```python
from build123d import *

# Parameters (mm, degrees)
BOSS_EXTRUDE1_DEPTH = 1.6


with BuildPart() as part:
    # Sketch1 → Boss-Extrude1 (new body)
    with BuildSketch(Plane(origin=(0, -12.08184695, 0), x_dir=(1, 0, 0), z_dir=(0, 1, 0))):
        with BuildLine():
            Line((7.068263687, 41.600601737), (-7.059496612, 41.600601737))
            ThreePointArc((-7.059496612, 41.600601737), (-8.738121808, 40.953226214), (-9.547386312, 39.346375699))
            add(Edge.make_bspline(
                [(-9.547386312, 39.346375699), (-9.791801042, 36.872209768), (-10.174780597, 34.427308106), (-11.191257392, 29.590412993), (-11.825986881, 27.198679788), (-13.350641046, 22.469109457), (-14.231234092, 20.161687267), (-16.219413971, 15.670679569), (-17.327255507, 13.484910955), (-19.77160384, 9.233454443), (-21.107913128, 7.167662826), (-23.287017843, 4.160685833), (-24.044102201, 3.171933948), (-25.600832941, 1.24516113), (-26.401965146, 0.30483539), (-30.518180843, -4.284811803), (-34.16377144, -7.599360565), (-38.1299904, -10.589142877)],
                knots=[0, 0, 0, 0, 0.125, 0.125, 0.25, 0.25, 0.375, 0.375, 0.5, 0.5, 0.625, 0.625, 0.6875, 0.6875, 0.75, 0.75, 1, 1, 1, 1], degree=3))
            ThreePointArc((-38.1299904, -10.589142877), (-39.094420308, -12.194619809), (-38.673009405, -14.019474345))
            ThreePointArc((-38.673009405, -14.019474345), (-38.081769626, -16.566513233), (-39.42061036, -18.812503006))
            ThreePointArc((-39.42061036, -18.812503006), (-40.390492541, -20.517035077), (-39.831968266, -22.396969027))
            add(Edge.make_bspline(
                [(-39.831968266, -22.396969027), (-38.283172708, -24.266437753), (-36.643071519, -26.058655413), (-33.174318098, -29.455880725), (-31.352030623, -31.054807711), (-29.43071323, -32.539448808)],
                knots=[0, 0, 0, 0, 0.5, 0.5, 1, 1, 1, 1], degree=3))
            add(Edge.make_bspline(
                [(-29.43071323, -32.539448808), (-27.320643605, -34.16992841), (-25.110907511, -35.649716155), (-20.460386406, -38.259954595), (-18.045119378, -39.375356082), (-14.281591244, -40.731351728), (-13.014141837, -41.126537478), (-10.462616624, -41.801653768), (-9.177088412, -42.082104136), (-5.291542564, -42.754094477), (-2.662588178, -42.976416738), (0.004383999, -42.976416738)],
                knots=[0, 0, 0, 0, 0.25, 0.25, 0.5, 0.5, 0.625, 0.625, 0.75, 0.75, 1, 1, 1, 1], degree=3))
            add(Edge.make_bspline(
                [(0.004383999, -42.976416738), (2.671656674, -42.976416738), (5.319285582, -42.754113953), (9.259525556, -42.067540092), (10.556225677, -41.781619701), (13.107012662, -41.101381696), (14.362802441, -40.706759914), (16.836410325, -39.811946458), (18.054248498, -39.311810579), (20.452976989, -38.208815379), (21.635192506, -37.605209835), (25.119535884, -35.649249598), (27.327228533, -34.170936704), (29.435499854, -32.542167102)],
                knots=[0, 0, 0, 0, 0.25, 0.25, 0.375, 0.375, 0.5, 0.5, 0.625, 0.625, 0.75, 0.75, 1, 1, 1, 1], degree=3))
            add(Edge.make_bspline(
                [(29.435499854, -32.542167102), (31.356661411, -31.057999079), (33.183178175, -29.455634698), (36.651766782, -26.058931244), (38.289020033, -24.270113959), (39.837842074, -22.401078618)],
                knots=[0, 0, 0, 0, 0.5, 0.5, 1, 1, 1, 1], degree=3))
            ThreePointArc((39.837842074, -22.401078618), (40.396592097, -20.52122374), (39.426929699, -18.816579853))
            ThreePointArc((39.426929699, -18.816579853), (38.088433126, -16.570796705), (38.67950123, -14.024082445))
            ThreePointArc((38.67950123, -14.024082445), (39.100802356, -12.199274218), (38.136401576, -10.593861236))
            add(Edge.make_bspline(
                [(38.136401576, -10.593861236), (34.168623759, -7.602959081), (30.509352448, -4.27682522), (26.366767099, 0.349726066), (25.563654335, 1.294607123), (24.01416015, 3.216210378), (23.26679186, 4.194046735), (21.106661228, 7.178559095), (19.77567512, 9.236115194), (17.332454935, 13.487332018), (16.22037441, 15.681088283), (14.719864957, 19.076008242), (14.246709963, 20.227996379), (13.365900278, 22.544460809), (12.957352394, 23.710625613), (11.82518653, 27.232396594), (11.194571791, 29.611161178), (10.183276163, 34.430925487), (9.800625177, 36.871434644), (9.556155738, 39.346351897)],
                knots=[0, 0, 0, 0, 0.25, 0.25, 0.3125, 0.3125, 0.375, 0.375, 0.5, 0.5, 0.625, 0.625, 0.6875, 0.6875, 0.75, 0.75, 0.875, 0.875, 1, 1, 1, 1], degree=3))
            ThreePointArc((9.556155738, 39.346351897), (8.746897744, 40.953218184), (7.068263687, 41.600601737))
        make_face()
        with BuildLine():
            ThreePointArc((2.917114338, 9.477212595), (2.756374668, 5.872981189), (3.951101823, 2.468726748))
            add(Edge.make_bspline(
                [(18.704113686, -16.363172993), (17.992145269, -15.660180667), (17.284020826, -14.953500566), (15.898077439, -13.511066303), (15.216988025, -12.778449721), (13.209804316, -10.545981706), (11.922619235, -9.014699706), (8.217020706, -4.29052926), (5.969838206, -0.988031562), (3.951101823, 2.468726748)],
                knots=[0, 0, 0, 0, 0.125, 0.125, 0.25, 0.25, 0.5, 0.5, 1, 1, 1, 1], degree=3))
            ThreePointArc((18.704113686, -16.363172993), (19.293025471, -17.93950559), (18.470275007, -19.407403142))
            add(Edge.make_bspline(
                [(-18.494716896, -19.382200256), (-18.156747928, -19.627153591), (-17.818664146, -19.871886584), (-17.13548839, -20.34790294), (-16.790775019, -20.579912893), (-15.746956693, -21.257369006), (-15.038196301, -21.684285132), (-12.870713002, -22.885961299), (-11.370716058, -23.581511117), (-9.025130071, -24.441385157), (-8.223466165, -24.698129558), (-6.613792479, -25.137565491), (-5.80401834, -25.321234472), (-3.359849379, -25.763841436), (-1.710600897, -25.914327465), (0.793635304, -25.91836178), (1.634808791, -25.88219159), (3.293827112, -25.736118011), (4.115824788, -25.626398759), (6.559865603, -25.190037003), (8.159961985, -24.756217145), (10.518010173, -23.899908948), (11.293937095, -23.580881464), (12.808242427, -22.888006864), (13.549502528, -22.513052805), (15.00267183, -21.710479018), (15.714628815, -21.282945031), (16.762116652, -20.60495391), (17.107865076, -20.372830636), (17.792765058, -19.896747026), (18.131563633, -19.652153318), (18.470275007, -19.407403142)],
                knots=[0, 0, 0, 0, 0.03125, 0.03125, 0.0625, 0.0625, 0.125, 0.125, 0.25, 0.25, 0.3125, 0.3125, 0.375, 0.375, 0.5, 0.5, 0.5625, 0.5625, 0.625, 0.625, 0.75, 0.75, 0.8125, 0.8125, 0.875, 0.875, 0.9375, 0.9375, 0.96875, 0.96875, 1, 1, 1, 1], degree=3))
            ThreePointArc((-18.494716896, -19.382200256), (-19.313315476, -17.938131693), (-18.759498896, -16.373291495))
            add(Edge.make_bspline(
                [(-4.019478984, 2.418815751), (-6.073388857, -1.004555589), (-8.371219964, -4.274194721), (-12.087144101, -8.96897705), (-13.369226154, -10.496572825), (-15.349259798, -12.736872688), (-16.018851728, -13.47516887), (-17.376233604, -14.935672121), (-18.066404983, -15.655773734), (-18.759498896, -16.373291495)],
                knots=[0, 0, 0, 0, 0.5, 0.5, 0.75, 0.75, 0.875, 0.875, 1, 1, 1, 1], degree=3))
            ThreePointArc((-4.019478984, 2.418815751), (-2.778667962, 5.846147783), (-2.919787203, 9.488441319))
            ThreePointArc((-2.919787203, 9.488441319), (0.005771232, 13.17752407), (2.917114338, 9.477212595))
        make_face(mode=Mode.SUBTRACT)
    extrude(amount=BOSS_EXTRUDE1_DEPTH)


solid = part.part
```
CAD build for the part. Positions are in the model's coordinates, mm. Round coordinates to 2 decimals unless told otherwise and drop trailing zeros. One line per question, with ' | ' between items.
Q1. Drop a flat-ended pin along its axis: pin 1 (7 mm diameter, centred on x = 0, z = -10.18, fed in from +Y). Give the stop position or say it passes through.
Completed:
pin 1: stops at y = -10.48
Q2. Probe probe 1 along Z at (x, y) = (0, -11.7); probe 2 along X at (y, z) = (-10.9, -11); probe 3 along Z at (x, y) = (1, -11.4). List the from-to ranges inside material, lowest first.
Completed:
probe 1: z = -41.6 to -13.18, 25.92 to 42.98 | probe 2: x = -18.76 to -2.89, 2.89 to 18.76 | probe 3: z = -41.6 to -13.01, 25.9 to 42.97
Q3. Two-plate mould, pull along X, no slides. Class faces 1 (the cylindrical face through (8.766, -11.293, -40.936)), 2 (the cylindrical face through (-0.07, -11.293, -13.177)), 3 (the cylindrical face through (-8.72, -11.29, -40.97)), 4 (the flat face through (8, -12.082, 0)): released by +X, released by -X, zero draft, split by the parting line, or undercut.
Completed:
face 1: released by +X | face 2: undercut | face 3: released by -X | face 4: zero draft
